Autodesk Inventor part; units mm, degrees
ref_plane "YZ Plane" through (0, 0, 0) normal (1, 0, 0) x (0, 1, 0)
ref_plane "XZ Plane" through (0, 0, 0) normal (0, 1, 0) x (-1, 0, 0)
ref_plane "XY Plane" through (0, 0, 0) normal (0, 0, 1) x (1, 0, 0)
sketch "Sketch1" plane through (0, 0, 0) normal (0, 0, 1) x (1, 0, 0)
  line L0 (-13.5, 24) -> (13.5, 24) construction
  line L1 (13.5, 24) -> (13.5, -24) construction
  line L2 (13.5, -24) -> (-13.5, -24) construction
  line L3 (-13.5, -24) -> (-13.5, 24) construction
  line L4 (-13.5, 0) -> (13.5, 0) construction
  line L5 (0, -24) -> (0, 24) construction
  circle A0 centre (0, 18.3) radius 2.75
  circle A1 centre (0, -18.3) radius 2.75
  line L6 (-60, 21.2) -> (-32, 21.2) construction
  line L7 (-32, 21.2) -> (-32, -25.8) construction
  line L8 (-32, -25.8) -> (-60, -25.8) construction
  line L9 (-60, -25.8) -> (-60, 21.2) construction
  line L10 (-46, 21.2) -> (-46, -25.8) construction
  line L11 (-60, -2.3) -> (-32, -2.3) construction
  circle A2 centre (-46, 15.7) radius 2.75
  circle A3 centre (-46, -20.3) radius 2.75
  circle A4 centre (46, 15.7) radius 2.75
  circle A5 centre (46, -20.3) radius 2.75
  line L12 (-82, 43.2) -> (82, 43.2)
  line L13 (82, 43.2) -> (82, -43.2)
  line L14 (82, -43.2) -> (-82, -43.2)
  line L15 (-82, -43.2) -> (-82, 43.2)
  point P0 (0, 0)
  point P1 (0, 0)
  dimension "d0" = 27
  dimension "d1" = 48
  dimension "d2" = 5.5
  dimension "d3" = 36.6
  dimension "d4" = 28
  dimension "d5" = 47
  dimension "d7" = 2.3
  dimension "d8" = 46
  dimension "d9" = 5.5
  dimension "d10" = 36
  dimension "d11" = 22
  dimension "d19" = 43.2
extrude "Extrusion1" add sketch "Sketch1" along normal blind 10
sketch "Sketch3" plane through (0, 0, 10) normal (0, 0, 1) x (1, 0, 0)
  line L0 (-82, 43.2) -> (-82, -43.2)
  line L1 (-82, -43.2) -> (82, -43.2)
  line L2 (-82, 43.2) -> (82, 43.2)
  line L3 (82, 43.2) -> (82, -43.2)
  line L4 (82, -43.2) -> (-82, -43.2)
  line L5 (-82, -43.2) -> (-82, 43.2)
  point P0 (0, 0)
extrude "Extrusion3" add sketch "Sketch3" along normal blind 90
sketch "Sketch4" plane through (-82, -43.2, 0) normal (-1, 0, 0) x (0, 0, 1)
  line L0 (0, 86.4) -> (0, 0)
  line L1 (0, 0) -> (100, 0)
  line L2 (100, 86.4) -> (100, 0)
  line L3 (0, 86.4) -> (100, 86.4)
  point P0 (0, 43.2)
extrude "Extrusion4" add sketch "Sketch4" along normal blind 10
sketch "Sketch5" plane through (-92, -43.2, 0) normal (-1, 0, 0) x (0, 0, 1)
  line L0 (0, 43.2) -> (100, 43.2) construction
  line L1 (100, 0) -> (100, 86.4) construction
  line L2 (0, 86.4) -> (100, 86.4) construction
  line L3 (50, 86.4) -> (50, 0) construction
  line L4 (0, 0) -> (100, 0) construction
  circle A0 centre (50, 43.2) radius 27.305
  dimension "d22" = 54.61
extrude "Extrusion5" add sketch "Sketch5" along normal blind 50
sketch "Sketch6" plane through (82, -43.2, 0) normal (0, -1, 0) x (1, 0, 0)
  line L0 (0, 0) -> (0, 100) construction
  line L1 (0, 50) -> (-174, 50) construction
  line L2 (-174, 100) -> (-174, 0) construction
  line L3 (-82, 0) -> (-82, 100) construction
  line L4 (0, 100) -> (-174, 100) construction
  circle A0 centre (-82, 50) radius 27.305
  dimension "d25" = 54.61
extrude "Extrusion6" add sketch "Sketch6" along normal blind 50
properties part number "aux_L"
The listing builds one solid part. Answer for the finished solid, in the listing's coordinates (mm). A direction names the side the tool comes from. Give positions to 0.01 mm unless a question says otherwise; leave off trailing zeros. Loops run counter-clockwise (first coordinate to the right, second up) from the corner with the lowest first, then second, coordinate; pieces in that order, holes last.
Item 1: A cutting plane is placed at B-B (y = 0). Give the vertices of the cut face in (x, z) (3 decimals), then the cut area to 3 significant figures.
Derived:
outline: (-142, 22.695) - (-92, 22.695) - (-92, 0) - (82, 0) - (82, 100) - (-92, 100) - (-92, 77.305) - (-142, 77.305) - close
area: 20,100 mm2
Item 2: Find the intervals of material crossed by line 1 along Y through (x, z) = (-46, 2); line 2 along Y through (x, z) = (0, 2); line 3 along X through (y, z) = (-20, 7), in increasing order.
Derived:
line 1: y = -43.2 to -23.05, -17.55 to 12.95, 18.45 to 43.2
line 2: y = -43.2 to -21.05, -15.55 to 15.55, 21.05 to 43.2
line 3: x = -92 to -48.73, -43.27 to -2.16, 2.16 to 43.27, 48.73 to 82
Item 3: A cutting plane is placed at C-C (z = 50). Give the vertices of the cut face in (x, y) (3 decimals), then the cut area to 3 significant figures.
Derived:
outline: (-142, -27.305) - (-92, -27.305) - (-92, -43.2) - (-27.305, -43.2) - (-27.305, -93.2) - (27.305, -93.2) - (27.305, -43.2) - (82, -43.2) - (82, 43.2) - (-92, 43.2) - (-92, 27.305) - (-142, 27.305) - close
area: 20,500 mm2
Item 4: Each of these flat-tipped pins is pushed along its axis until it touches: pin 1 Ø5 at (x, y) = (-46, 15.7) entering from -Z; pin 2 Ø8 at (x, z) = (-114, 72.5) entering from +Y. Where does it stop, or does it pass through?
Derived:
pin 1: stops at z = 10
pin 2: stops at y = 20.08
Item 5: A cutting plane is placed at D-D (x = 46). Give the vertices of the cut face in (y, z).
Derived:
outline: (-43.2, 0) - (-23.05, 0) - (-23.05, 10) - (-17.55, 10) - (-17.55, 0) - (12.95, 0) - (12.95, 10) - (18.45, 10) - (18.45, 0) - (43.2, 0) - (43.2, 100) - (-43.2, 100) - close
Item 6: A cutting plane is placed at A-A (x = 0). Give the vertices of the cut face in (y, z) (3 decimals).
Derived:
outline: (-93.2, 22.695) - (-43.2, 22.695) - (-43.2, 0) - (-21.05, 0) - (-21.05, 10) - (-15.55, 10) - (-15.55, 0) - (15.55, 0) - (15.55, 10) - (21.05, 10) - (21.05, 0) - (43.2, 0) - (43.2, 100) - (-43.2, 100) - (-43.2, 77.305) - (-93.2, 77.305) - close
Item 7: A tool of negligible diameter and unlimited length cuts with its end or side. For faces 1 (the flat face through (0, -18, 10)), 2 (the cylindrical face through (-116.65, -23.024, 64.679)), 3 (the flat face through (-142, 0, 50)), from which of +Z, -Z, +X, -X, +Y, -Y can it reach the whole face along a straight path? Write none if from no direction.
Derived:
face 1: -Z
face 2: -X
face 3: +Z, -Z, -X, +Y, -Y
Item 8: Determine the mould class of faces 4 (the cylindrical face through (-48.747, 15.579, 4.93)), 5 (the cylindrical face through (-3.555, -67.85, 22.927)), 6 (the flat face through (-92, 29, 49)), 7 (the flat face through (0, -93.2, 50)) for opening direction X: +X half, -X half, draft (parallel to the pull), parting line (faces both ways), or undercut.
Derived:
face 4: undercut
face 5: parting line
face 6: -X half
face 7: draft
